Check sheet for the modelled part. Datum: model origin and axes. Units: mm. Round coordinates to 2 decimals unless told otherwise and drop trailing zeros. Order: outer loops, then holes, each group sorted by start corner. A loop starts at its lowest first (then second) coordinate and runs counter-clockwise, first axis right, second up. Notation, with made-up numbers: (50, 15) -> (87, 15) arc R24 cw to (87, 41) -> close; hole circle Ø9 at (73.5, -17.5). An arc over 180 degrees is marked (long way). Use CSV: the item, a comma, the result in double quotes.
```python
from build123d import *

# Parameters (mm, degrees)
SKETCH1_R           = 1.5
SKETCH1_W           = 73
SKETCH1_H           = 26
BOSS_EXTRUDE1_DEPTH = 3


with BuildPart() as part:
    # Sketch1 → Boss-Extrude1 (new body)
    with BuildSketch(Plane.XY):
        Polygon((-40, -91), (-15, -91), (-15, -75), (112, -75), (112, -73), (122, -73), (122, -91), (140, -91), (140, -57), (127, -57), (127, 1), (140, 1), (140, 23), (-9, 23), (-9, 9), (-40, 9), align=None)
        with Locations((-5, 9)):
            Circle(SKETCH1_R, mode=Mode.SUBTRACT)
        with Locations((136, 9)):
            Circle(SKETCH1_R, mode=Mode.SUBTRACT)
        with Locations((136, -87)):
            Circle(SKETCH1_R, mode=Mode.SUBTRACT)
        with Locations((-36, -87)):
            Circle(SKETCH1_R, mode=Mode.SUBTRACT)
        with Locations((32, -16)):
            Rectangle(SKETCH1_W, SKETCH1_H, mode=Mode.SUBTRACT)
    extrude(amount=-BOSS_EXTRUDE1_DEPTH)


solid = part.part
```
Q1. Sectioned sample at C-C, the plane x = 118. Enter the section's corners in (y, z), then the cut area to 3 significant figures.
Result sheet:
outline,"(-73, -3) -> (23, -3) -> (23, 0) -> (-73, 0) -> close"
area,"288 mm^2"
Q2. Sectioned sample at A-A, the plane x = 18. Enter the section's corners in (y, z), then the cut area to 3 significant figures.
Result sheet:
outline,"(-75, -3) -> (-29, -3) -> (-29, 0) -> (-75, 0) -> close; (-3, -3) -> (23, -3) -> (23, 0) -> (-3, 0) -> close"
area,"216 mm^2"
Q3. Scan lines: L1, parallel to Y at x = 136, z = -1.2; L2, parallel to X at y = -87, z = -2.4; L3, parallel to Y at x = 128, z = -0.25. Record each from-to range of solid material in increasing order.
Result sheet:
L1,"y = -91 to -88.5, -85.5 to -57, 1 to 7.5, 10.5 to 23"
L2,"x = -40 to -37.5, -34.5 to -15, 122 to 134.5, 137.5 to 140"
L3,"y = -91 to -57, 1 to 23"
Q4. Sectioned sample at D-D, the plane y = -38. Enter the section's corners in (x, z).
Result sheet:
outline,"(-40, -3) -> (127, -3) -> (127, 0) -> (-40, 0) -> close"
Q5. Sectioned sample at B-B, the plane z = -1.6. Enter the section's corners in (x, y), then the cut area to 3 significant figures.
Result sheet:
outline,"(-40, -91) -> (-15, -91) -> (-15, -75) -> (112, -75) -> (112, -73) -> (122, -73) -> (122, -91) -> (140, -91) -> (140, -57) -> (127, -57) -> (127, 1) -> (140, 1) -> (140, 23) -> (-9, 23) -> (-9, 9) -> (-40, 9) -> close; hole circle Ø3 at (-36, -87); hole circle Ø3 at (-5, 9); hole (-4.5, -29) -> (68.5, -29) -> (68.5, -3) -> (-4.5, -3) -> close; hole circle Ø3 at (136, -87); hole circle Ø3 at (136, 9)"
area,"15,200 mm^2"
Q6. Go/stop test with flat-tipped pins: pin 1 (2.5 mm diameter, centred on x = 136, y = 9, fed in from -Z); pin 2 (4 mm diameter, centred on x = 136, y = -87, fed in from -Z); pin 3 (0.9 mm diameter, centred on y = 14, z = -1.5, fed in from -X); pin 4 (1.5 mm diameter, centred on x = -24.5, z = -1.5, fed in from +Y). Record where each tip stops, or that it passes through.
Result sheet:
pin 1,"passes through"
pin 2,"stops at z = -3"
pin 3,"stops at x = -9"
pin 4,"stops at y = 9"
